Here's the drawing with two shaded views (mm, measured from the low corner). I have some questions. A direction names the side the tool comes from. Coordinates: 2 decimals unless noted, no trailing zeros. Write each loop counter-clockwise with the first axis right and the second up, starting at its lowest first coordinate (ties: lowest second). Pieces come first, ordered by that corner, then holes. Notation, with made-up numbers: (-29.5, -28.75) -> (15.5, -28.75) arc R27 cw to (15.5, -11.75) -> close; hole circle Ø10 at (-38, 83). An arc over 180 degrees is marked (long way). Put each result on its own line as item: value.
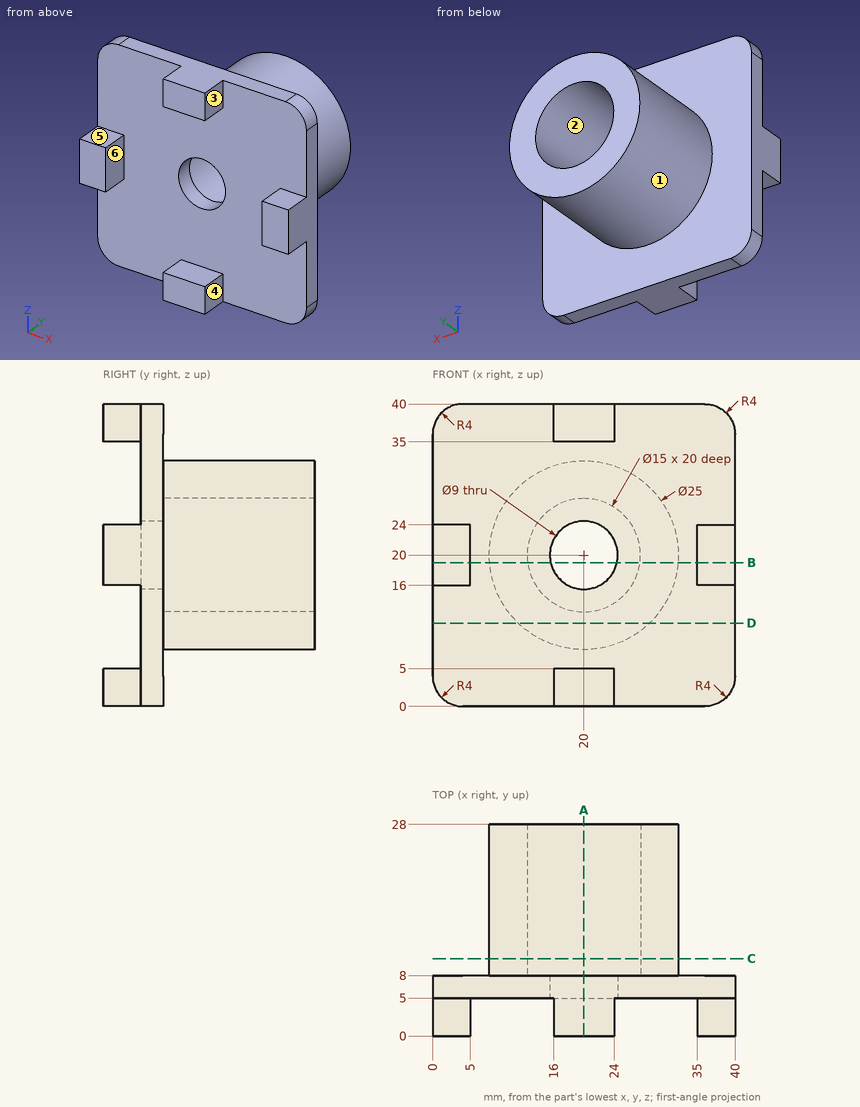
Item 1: Imagine slicing it at D-D on z = 11. Write out the boundary of the cut face in (x, y).
Output:
outline: (0, 5) -> (40, 5) -> (40, 8) -> (28.67, 8) -> (28.67, 28) -> (11.33, 28) -> (11.33, 8) -> (0, 8) -> close
Item 2: Imagine slicing it at B-B on z = 19. Write out the boundary of the cut face in (x, y), then the cut area to 3 significant figures.
Output:
outline: (0, 0) -> (5, 0) -> (5, 5) -> (15.61, 5) -> (15.61, 8) -> (12.57, 8) -> (12.57, 28) -> (7.54, 28) -> (7.54, 8) -> (0, 8) -> close; (24.39, 5) -> (35, 5) -> (35, 0) -> (40, 0) -> (40, 8) -> (32.46, 8) -> (32.46, 28) -> (27.43, 28) -> (27.43, 8) -> (24.39, 8) -> close
area: 345 mm²
Item 3: For P1, Ø20, axis at x = 20.5, z = 27, coming from the +Y side; P2, Ø4, axis at y = 2, z = 37, coming from the +X side; P3, Ø2.5, axis at x = 3.5, y = 1.5, coming from the +Z side; P4, Ø12, axis at y = 23.5, z = 11, coming from the -X side, each with a flat end and sliding along its axis, tell me the tip position at first contact or that it passes through.
Output:
P1: stops at y = 28
P2: stops at x = 24
P3: stops at z = 24
P4: stops at x = 7.87
Item 4: Please list where these lines run through material, in increasing order: line 1 along Z through (x, y) = (20, 6.75); line 2 along Y through (x, z) = (34, 22). Write a range as from..to.
Output:
line 1: z = 0..15.5, 24.5..40
line 2: y = 5..8
Item 5: Imagine slicing it at A-A on x = 20. Write out the boundary of the cut face in (y, z).
Output:
outline: (0, 0) -> (8, 0) -> (8, 7.5) -> (28, 7.5) -> (28, 12.5) -> (8, 12.5) -> (8, 15.5) -> (5, 15.5) -> (5, 5) -> (0, 5) -> close; (0, 35) -> (5, 35) -> (5, 24.5) -> (8, 24.5) -> (8, 27.5) -> (28, 27.5) -> (28, 32.5) -> (8, 32.5) -> (8, 40) -> (0, 40) -> close
Item 6: If we mould it in two halves opening along Z, with no side actions, what happens to the marked faces 1, 2 and 3? For each: released by +Z, released by -Z, zero draft, split by the parting line, or undercut.
Output:
face 1: split by the parting line
face 2: undercut
face 3: zero draft
Item 7: Imagine slicing it at C-C on y = 10.25. Write out the boundary of the cut face in (x, z), then the cut area to 3 significant figures.
Output:
outline: circle Ø25 at (20, 20); hole circle Ø15 at (20, 20)
area: 314 mm²
Item 8: Which directions (+Z, -Z, +X, -X, +Y, -Y) give clear straight access to the entire face, cutting with the end or side of a thin tool? Please do the marked faces 4, 5 and 6.
Output:
face 4: +Z, -Z, +X, -Y
face 5: +Z, +X, -X, -Y
face 6: +Z, -Z, -Y
